```python
from build123d import *

# Parameters (mm, degrees)
F0_R     = 25
F2_DEPTH = 5
F1_W     = 15
F1_H     = 10
F3_DEPTH = 40
F4_W     = 5
F4_H     = 10
F5_DEPTH = 25
F6_R     = 2.5
F7_DEPTH = 32.501
F8_R     = 4.99999


# Not quite as in the source:
# - a fillet or chamfer is up to 0.001 mm smaller than in the source, because OpenCascade refuses the exact size


with BuildPart() as f2:
    # F0 (on Top) → F2 (new body)
    with BuildSketch(Plane.XY):
        Circle(F0_R)
    extrude(amount=F2_DEPTH)

    # F1 (on Top) → F3 (join)
    with BuildSketch(Plane.XY):
        Rectangle(F1_W, F1_H)
    extrude(amount=F3_DEPTH)

    # F4 (on face) → F5 (cut)
    with BuildSketch(Plane.XY.offset(40)):
        Rectangle(F4_W, F4_H)
    extrude(amount=-F5_DEPTH, mode=Mode.SUBTRACT)

    # F6 (on face) → F7 (cut, through all)
    with BuildSketch(Plane.YZ.offset(7.5)):
        with Locations((0, 35)):
            Circle(F6_R)
    extrude(amount=-F7_DEPTH, mode=Mode.SUBTRACT)

    # F8 (radius 5 in the source; OpenCascade refuses exactly that, so slightly less here)
    f8_edges = [f2.edges().sort_by_distance(p)[0] for p in [
        (-5, 5, 40),
        (-5, -5, 40),
        (5, 5, 40),
        (5, -5, 40),
    ]]
    fillet(f8_edges, radius=F8_R)


solid = f2.part
```
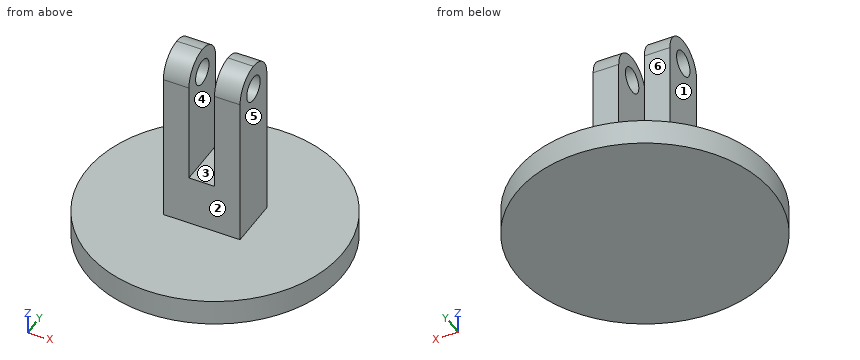
The model under review builds one solid part; all positions refer to its coordinate system, in mm. Face numbers are marked on the shaded views. A direction names the side the tool comes from. Give positions to 0.01 mm unless a question says otherwise; leave off trailing zeros. Write each loop counter-clockwise with the first axis right and the second up, starting at its lowest first coordinate (ties: lowest second). Pieces come first, ordered by that corner, then holes.
(1) Consider section D-D, the plane y = 3.5. Give the boundary of the cut face in (x, z), and give its area (3 significant figures).
(2) To check wall thickness, follow L1, parallel to Z at x = -4.05, y = 0; L2, parallel to Z at x = 12.5, y = 8; L3, parallel to Z at x = 4.5, y = 1.5. State the ranges of each line that lie inside material, in increasing order.
(3) For P1, Ø8, axis at y = 0.5, z = 25.5, coming from the -X side; P2, Ø8, axis at x = -3, z = 27.5, coming from the -Y side; P3, Ø5, axis at y = 2, z = 29.5, coming from the +X side; P4, Ø4.5, axis at y = 0, z = 35, coming from the -X side, all flat-tipped, find the tip position at first contact; note any pin that passes through.
(4) Tool access review of the marked faces 4, 5 and 6: name each direction out of +Z, -Z, +X, -X, +Y, -Y from which nothing blocks a thin tool from reaching the whole face with its end or side.
(5) Consider section B-B, the plane x = 0. Give the boundary of the cut face in (y, z), and give its area (3 significant figures).
(6) The part is to be moulded in two halves that separate along X. For the marked faces 1, 2 and 3, say which applies: released by +X, released by -X, zero draft, split by the parting line, or undercut.
(7) Consider section A-A, the plane z = 17. Give the boundary of the cut face in (x, y).
Returned:
1. outline: (-24.75, 0) - (24.75, 0) - (24.75, 5) - (7.5, 5) - (7.5, 38.57) - (2.5, 38.57) - (2.5, 15) - (-2.5, 15) - (-2.5, 38.57) - (-7.5, 38.57) - (-7.5, 5) - (-24.75, 5) - close
1. area: 633 mm2
2. L1: z = 0 to 32.5, 37.5 to 40
2. L2: z = 0 to 5
2. L3: z = 0 to 33, 37 to 39.77
3. P1: stops at x = -7.5
3. P2: stops at y = -5
3. P3: stops at x = 7.5
3. P4: passes through
4. face 4: +Z, +Y, -Y
4. face 5: +Z, +X, +Y, -Y
4. face 6: +Z, +X, -X, +Y
5. outline: (-25, 0) - (25, 0) - (25, 5) - (5, 5) - (5, 15) - (-5, 15) - (-5, 5) - (-25, 5) - close
5. area: 350 mm2
6. face 1: released by -X
6. face 2: zero draft
6. face 3: undercut
7. outline: (-7.5, -5) - (-2.5, -5) - (-2.5, 5) - (-7.5, 5) - close; (2.5, -5) - (7.5, -5) - (7.5, 5) - (2.5, 5) - close
